Model file for the job. Use its own axes, mm. Give positions to 0.01 mm unless a question says otherwise; leave off trailing zeros. Write each loop counter-clockwise with the first axis right and the second up, starting at its lowest first coordinate (ties: lowest second). Pieces come first, ordered by that corner, then holes. Notation, with made-up numbers: M 83.5,71 L 100.5,71 A14 cw 100.5,87 Z; hole C 4.5,71.5 d3. An arc over 180 degrees is marked long. Answer as a JSON object with one key per item and string values. Group by question number.
```python
from build123d import *

# Parameters (mm, degrees)
BOSS_EXTRUDE1_DEPTH = 3.048
HOLE1_D             = 3.81
HOLE1_DEPTH         = 15.24
LPATTERN1_COUNT     = 4
LPATTERN1_PITCH     = 80.01


with BuildPart() as part:
    # Sketch1 → Boss-Extrude1 (new, symmetric)
    with BuildSketch(Plane.XY):
        Polygon((-59.885399579, 149.447165674), (-298.958, 0), (0, 0), (88.196600421, 149.447165674), align=None)
    extrude(amount=BOSS_EXTRUDE1_DEPTH, both=True)

    # Hole1
    with Locations(Plane.XY.offset(3.048)):
        with Locations((-258.826, 6.096)):
            hole1 = Hole(HOLE1_D / 2, depth=HOLE1_DEPTH)

    # LPattern1: Hole1 ×4
    with Locations(*[(i * LPATTERN1_PITCH, 0, 0) for i in range(1, LPATTERN1_COUNT)]):
        add(hole1, mode=Mode.SUBTRACT)


solid = part.part
```
Q1. Slice it at A-A, the plane z = -2. Write the cut outline in (x, y) (3 decimals), then the cut area to 3 significant figures.
Q2. Wall check: L1, parallel to Y at x = -268.5, z = -2; L2, parallel to Y at x = 65, z = 2.5; L3, parallel to X at y = 110, z = 0.75. Give the ranges that are in metal, low to high.
Q3. Drop flat-ended pins along their axis: P1, Ø1, axis at y = 31.5, z = 0, coming from the -X side; P2, Ø2.5, axis at x = -258.826, y = 6.096, coming from the -Z side. Give the stop position or say it passes through.
Q4. Slice it at C-C, the plane y = 115.5. Write the cut outline in (x, z).
Q5. Slice it at B-B, the plane x = 4.5. Write the cut outline in (y, z), then the cut area to 3 significant figures.
Solved:
{
 "1": {"outline": "M -298.958,0 L 0,0 L 88.197,149.447 L -59.885,149.447 Z; hole C -258.826,6.096 d3.81; hole C -178.816,6.096 d3.81; hole C -98.806,6.096 d3.81; hole C -18.796,6.096 d3.81", "area": "33,400 mm²"},
 "2": {"L1": "y = 0 to 19.04", "L2": "y = 110.14 to 149.45", "L3": "x = -122.99 to 64.92"},
 "3": {"P1": "stops at x = -249.37", "P2": "passes through"},
 "4": {"outline": "M -114.19,-3.05 L 68.16,-3.05 L 68.16,3.05 L -114.19,3.05 Z"},
 "5": {"outline": "M 7.63,-3.05 L 149.45,-3.05 L 149.45,3.05 L 7.63,3.05 Z", "area": "865 mm²"}
}
